Read the model definition and answer for the solid it produces. Units are mm, in the model's axes. A direction names the side the tool comes from. Coordinates: 2 decimals unless noted, no trailing zeros. Loops run counter-clockwise (first coordinate to the right, second up) from the corner with the lowest first, then second, coordinate; pieces in that order, holes last. Notation, with made-up numbers: (-5, 11.25) - (13, 11.25) arc R16 cw to (13, 38.25) - close; hole circle Ø6 at (-22.5, 53). An arc over 180 degrees is marked (long way). One line per question, with ' | ' between items. Start each with the question number.
```python
from build123d import *

# Parameters (mm, degrees)
SKETCH_1_W               = 77
SKETCH_1_H               = 10
EXTRUDE_1_DEPTH          = 55
CUT_EXTRUDE_1_DEPTH      = 639.884201719
SKETCH_4_W               = 15
SKETCH_4_H               = 20
CUT_EXTRUDE_3_DEPTH      = 10
SKETCH_5_W               = 19.997544879
SKETCH_5_H               = 6
EXTRUDE_2_DEPTH          = 26
SKETCH_8_R               = 5
CUT_EXTRUDE_4_DEPTH      = 409.554479516
CUT_EXTRUDE_5_DEPTH      = 407.529462179
CUT_EXTRUDE_5_DEPTH_BACK = 407.529462179
SKETCH_10_R              = 4


with BuildPart() as part:
    # 草图1 → 凸台-拉伸1 (new body)
    with BuildSketch(Plane.ZY.offset(242.287512766)):
        with Locations((526.914147293, -246.15455511)):
            Rectangle(SKETCH_1_W, SKETCH_1_H)
    extrude(amount=EXTRUDE_1_DEPTH)

    # 草图2 → 切除-拉伸1 (cut, through all)
    with BuildSketch(Plane(origin=(0, -241.15455511, 0), x_dir=(1, 0, 0), z_dir=(0, 1, 0))):
        with BuildLine():
            Line((-242.287512766, -506.914147293), (-242.287512766, -488.414147293))
            Line((-242.287512766, -488.414147293), (-297.287512766, -488.414147293))
            Line((-297.287512766, -488.414147293), (-297.287512766, -501.914147293))
            add(Edge.make_bspline(
                [(-242.287512766, -506.914147293), (-271.288122088, -514.395388486), (-297.287512766, -501.914147293)],
                knots=[0, 0, 0, 1, 1, 1], degree=2))
        make_face()
        with BuildLine():
            Line((-242.287512766, -546.914147293), (-242.287512766, -565.414147293))
            Line((-242.287512766, -565.414147293), (-297.287512766, -565.414147293))
            Line((-297.287512766, -565.414147293), (-297.287512766, -551.914147293))
            add(Edge.make_bspline(
                [(-242.287512766, -546.914147293), (-271.288122088, -539.4329061), (-297.287512766, -551.914147293)],
                knots=[0, 0, 0, 1, 1, 1], degree=2))
        make_face()
    extrude(amount=-CUT_EXTRUDE_1_DEPTH, mode=Mode.SUBTRACT)

    # 草图4 → 切除-拉伸3 (cut)
    with BuildSketch(Plane.XZ.offset(251.15455511)):
        Polygon((-242.287512766, 517.028807482), (-242.287512766, 526.914147293), (-242.287512766, 536.914147293), (-262.287512766, 536.914147293), (-262.287512766, 516.914147293), align=None)
        with Locations((-289.787512766, 526.914147293)):
            Rectangle(SKETCH_4_W, SKETCH_4_H)
    extrude(amount=-CUT_EXTRUDE_3_DEPTH, mode=Mode.SUBTRACT)

    # 草图5 → 凸台-拉伸2 (add)
    with BuildSketch(Plane.XZ.offset(251.15455511)):
        Polygon((-262.287512766, 537.414147293), (-282.285057645, 537.414147293), (-282.287512766, 543.414147293), (-262.287512766, 543.414147293), align=None)
        with Locations((-272.286285206, 513.414147293)):
            Rectangle(SKETCH_5_W, SKETCH_5_H)
    extrude(amount=EXTRUDE_2_DEPTH)

    # 草图8 → 切除-拉伸4 (cut, through all)
    with BuildSketch(Plane.XY.offset(543.414147293)):
        with Locations((-272.287512766, -266.15455511)):
            Circle(SKETCH_8_R)
        with BuildLine():
            Line((-262.287512766, -266.15455511), (-262.287512766, -277.15455511))
            Line((-262.287512766, -277.15455511), (-282.287512766, -277.15455511))
            Line((-282.287512766, -277.15455511), (-282.287512766, -266.15455511))
            ThreePointArc((-282.287512766, -266.15455511), (-272.287512766, -276.15455511), (-262.287512766, -266.15455511))
        make_face()
    extrude(amount=-CUT_EXTRUDE_4_DEPTH, mode=Mode.SUBTRACT)

    # 草图10 → 切除-拉伸5 (cut, two sides: drawn at the far end of the back side and taken through both)
    with BuildSketch(Plane(origin=(0, 0, 526.914147293), x_dir=(-1, 0, 0), z_dir=(0, 0, -1)).offset(-CUT_EXTRUDE_5_DEPTH_BACK)):
        with Locations((295.287512766, -246.15455511)):
            Circle(SKETCH_10_R)
    extrude(amount=CUT_EXTRUDE_5_DEPTH + CUT_EXTRUDE_5_DEPTH_BACK, mode=Mode.SUBTRACT)


solid = part.part
```
1) Given pin 1 Ø3 at (x, y) = (-253.5, -248) entering from -Z; pin 2 Ø8 at (x, y) = (-272.29, -266.15) entering from +Z; pin 3 Ø10 at (x, y) = (-270, -266.5) entering from +Z; pin 4 Ø5 at (y, z) = (-245.5, 530.5) entering from +X, each flat-ended and moving along its own axis, determine where each tip first touches the part or whether it passes through.
2) The mould has two halves that part along X. Classify faces 1 (the cylindrical face through (-291.29, -246.04, 542.85)), 2 (the flat face through (-242.288, -246, 512)), 3 (the flat face through (-272, -261, 510.414)): released by +X, released by -X, zero draft, split by the parting line, or undercut.
3) The part is cut by section B-B on z = 515. Write down the section's boundary in (x, y), and give its area (3 significant figures).
4) The part is cut by section A-A on y = -254. Write down the section's boundary in (x, z), and give its area (3 significant figures).
5) Find the intervals of material crossed by line 1 along Z through (x, y) = (-271.5, -255); line 2 along Y through (x, z) = (-268, 531); line 3 along X through (y, z) = (-259.5, 516), in increasing order. Write a range as from..to.
6) The part is cut by section D-D on z = 527. Write down the section's boundary in (x, y), and give its area (3 significant figures).
7) The part is cut by section C-C on y = -269. Write down the section's boundary in (x, z).
8) Which of the six approach directions +Z, -Z, +X, -X, +Y, -Y give full straight-line access (tool end or side, diameter ignored) to faces 4 (the flat face through (-272, -261, 516.414)), 5 (the flat face through (-262.288, -259, 540)), 6 (the cylindrical face through (-275.973, -262.775, 540.456))?
Answer below:
1) pin 1: z = 508.87 | pin 2: through | pin 3: z = 543.41 | pin 4: x = -262.29
2) face 1: undercut | face 2: released by +X | face 3: zero draft
3) outline: (-297.29, -251.15) - (-282.29, -251.15) - (-282.29, -266.38) arc R10 ccw to (-262.29, -266.15) - (-262.29, -251.15) - (-242.29, -251.15) - (-242.29, -241.15) - (-297.29, -241.15) - (-297.29, -242.69) arc R4 cw (long way) to (-297.29, -249.62) - close; hole circle Ø10 at (-272.29, -266.15) | area: 888 mm2
4) outline: (-282.29, 510.41) - (-262.29, 510.41) - (-262.29, 516.41) - (-282.29, 516.41) - close; (-282.29, 537.41) - (-262.29, 537.41) - (-262.29, 543.41) - (-282.29, 543.41) - close | area: 240 mm2
5) line 1: 510.41..516.41, 537.41..543.41 | line 2: -251.15..-241.15 | line 3: -282.29..-262.29
6) outline: (-282.29, -251.15) - (-262.29, -251.15) - (-262.29, -241.15) - (-282.29, -241.15) - close | area: 200 mm2
7) outline: (-281.87, 510.41) - (-276.4, 510.41) - (-276.4, 516.41) - (-281.87, 516.41) - close; (-281.87, 537.41) - (-276.4, 537.41) - (-276.4, 543.41) - (-281.87, 543.41) - close; (-268.18, 510.41) - (-262.7, 510.41) - (-262.7, 516.41) - (-268.18, 516.41) - close; (-268.18, 537.41) - (-262.7, 537.41) - (-262.7, 543.41) - (-268.18, 543.41) - close
8) face 4: +X, -X, -Y | face 5: +Z, -Z, +X, -Y | face 6: +Z, -Z
